Geometry check sheet. Reference: the model listing, model coordinates, mm. Coordinates: 2 decimals unless noted, no trailing zeros. Write each loop counter-clockwise with the first axis right and the second up, starting at its lowest first coordinate (ties: lowest second). Pieces come first, ordered by that corner, then holes. Notation, with made-up numbers: (56.25, 9) - (97.25, 9) arc R30 cw to (97.25, 43) - close; hole circle Ø9 at (89, 88.25). An arc over 180 degrees is marked (long way). Answer as a JSON object with one key per item and string values. Group by question number.
from build123d import *

# Parameters (mm, degrees)
CROQUIS1_W                         = 50
CROQUIS1_H                         = 15
CROQUIS1_R                         = 1.35
CROQUIS1_R_2                       = 1.39
CROQUIS1_R_3                       = 1.4
CROQUIS1_R_4                       = 1.41
CROQUIS1_R_5                       = 1.42
CROQUIS1_R_6                       = 1.43
CROQUIS1_R_7                       = 1.44
CROQUIS1_R_8                       = 1.45
SALIENTE_EXTRUIR1_DEPTH            = 3
TALADRO_DE_MARGEN_PARA_M2_51_D     = 3.1
TALADRO_DE_MARGEN_PARA_M2_51_DEPTH = 3.18
TALADRO_DE_MARGEN_PARA_M2_51_TIP   = 0.931333959


with BuildPart() as part:
    # Croquis1 → Saliente-Extruir1 (new body)
    with BuildSketch(Plane(origin=(0, 0, 0), x_dir=(1, 0, 0), z_dir=(0, 1, 0))):
        Rectangle(CROQUIS1_W, CROQUIS1_H)
        with Locations(Location((-21.662668198, 0, 0), (0, 0, 270))):
            Circle(CROQUIS1_R, mode=Mode.SUBTRACT)
        with Locations(Location((-15.977400582, 0, 0), (0, 0, 270))):
            Circle(CROQUIS1_R_2, mode=Mode.SUBTRACT)
        with Locations(Location((-10.330808256, 0, 0), (0, 0, 270))):
            Circle(CROQUIS1_R_3, mode=Mode.SUBTRACT)
        with Locations(Location((-5.032293538, 0, 0), (0, 0, 270))):
            Circle(CROQUIS1_R_4, mode=Mode.SUBTRACT)
        with Locations(Location((0, 0, 0), (0, 0, 270))):
            Circle(CROQUIS1_R_5, mode=Mode.SUBTRACT)
        with Locations(Location((5.626588796, 0, 0), (0, 0, 270))):
            Circle(CROQUIS1_R_6, mode=Mode.SUBTRACT)
        with Locations(Location((11.516395661, 0, 0), (0, 0, 270))):
            Circle(CROQUIS1_R_7, mode=Mode.SUBTRACT)
        with Locations(Location((16.88744942, 0, 0), (0, 0, 270))):
            Circle(CROQUIS1_R_8, mode=Mode.SUBTRACT)
    extrude(amount=SALIENTE_EXTRUIR1_DEPTH)

    # Taladro de margen para M2.51
    with Locations(Plane(origin=(0, 3, 0), x_dir=(1, 0, 0), z_dir=(0, 1, 0))):
        with Locations((22.148927614, 0)):
            Hole(TALADRO_DE_MARGEN_PARA_M2_51_D / 2, depth=TALADRO_DE_MARGEN_PARA_M2_51_DEPTH)
            with Locations((0, 0, -(TALADRO_DE_MARGEN_PARA_M2_51_DEPTH + TALADRO_DE_MARGEN_PARA_M2_51_TIP / 2))):  # 118° drill point
                Cone(0, TALADRO_DE_MARGEN_PARA_M2_51_D / 2, TALADRO_DE_MARGEN_PARA_M2_51_TIP, mode=Mode.SUBTRACT)


solid = part.part
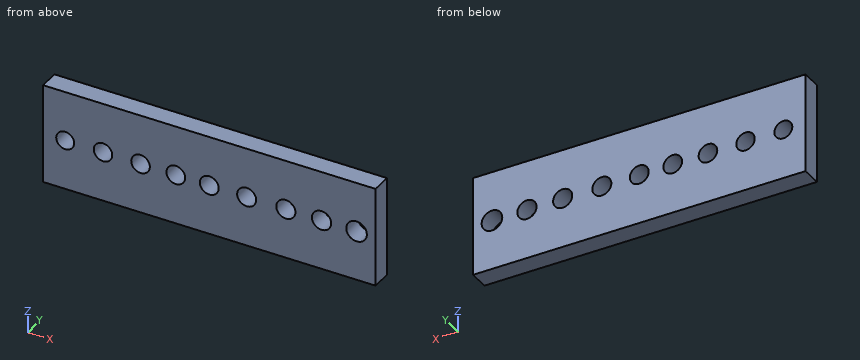
(1) Section check A-A (x = 0). Record the cut outline in (y, z).
(2) Gauge pin test, flat ends, axial feed: pin 1 (2 mm diameter, centred on x = -15.98, z = 0, fed in from +Y); pin 2 (5 mm diameter, centred on x = 22.15, z = 0, fed in from -Y). Record the tip position at first contact, or that the pin passes through.
(3) Section check D-D (x = 5). Record the cut outline in (y, z), and give its area (3 significant figures).
(4) Material ranges on L1, parallel to Z at x = -10, y = 0.45; L2, parallel to Z at x = 22, y = 1.8, recorded low to high. Write a range as [from, to].
(5) Section check B-B (z = 0). Count the separate pieces of the cut face and the enclosed holes in it, and give its area (3 significant figures).
Conclusion:
{
 "1": {"outline": "(0, -7.5) - (3, -7.5) - (3, -1.42) - (0, -1.42) - close; (0, 1.42) - (3, 1.42) - (3, 7.5) - (0, 7.5) - close"},
 "2": {"pin 1": "passes through", "pin 2": "stops at y = 0"},
 "3": {"outline": "(0, -7.5) - (3, -7.5) - (3, -1.29) - (0, -1.29) - close; (0, 1.29) - (3, 1.29) - (3, 7.5) - (0, 7.5) - close", "area": "37.3 mm^2"},
 "4": {"L1": "z = [-7.5, -1.36], [1.36, 7.5]", "L2": "z = [-7.5, -1.54], [1.54, 7.5]"},
 "5": {"separate pieces": "10", "enclosed holes": "0", "area": "73.0 mm^2"}
}
